Read the model definition and answer for the solid it produces. Units are mm, in the model's axes. Coordinates: 2 decimals unless noted, no trailing zeros. Write each loop counter-clockwise with the first axis right and the second up, starting at its lowest first coordinate (ties: lowest second). Pieces come first, ordered by that corner, then holes.
(1) The part is cut by section B-B, the plane y = 46. Determine the outline of the cut face in (x, z) (3 decimals).
(2) Straight lines are drawn through the part: line 1 along Z through (x, y) = (0.55, 61) (3 decimals); line 2 along Z through (x, y) = (1.45, 25.5); line 3 along Y through (x, z) = (2.9, 21). For each, find the intervals that lie inside material, in ascending order.
(3) The part is cut by section A-A, the plane y = 35. Determine the outline of the cut face in (x, z), and give its area (3 significant figures).
(4) Given pin 1 (1.5 mm diameter, centred on x = 2, z = 8.5, fed in from +Y); pin 2 (1 mm diameter, centred on x = 2.5, z = 187, fed in from -Y) (3 decimals); pin 3 (1.5 mm diameter, centred on x = 2, z = 198, fed in from -Y), each flat-ended and moving along its own axis, determine where each tip first touches the part or whether it passes through.
(5) The part is cut by section C-C, the plane x = 2.25. Determine the outline of the cut face in (y, z) (3 decimals).
(6) The part is cut by section D-D, the plane z = 59.5. Determine the outline of the cut face in (x, y).
Autodesk Inventor part; units mm, degrees
ref_plane "YZ Plane" through (0, 0, 0) normal (1, 0, 0) x (0, 1, 0)
ref_plane "XZ Plane" through (0, 0, 0) normal (0, 1, 0) x (-1, 0, 0)
ref_plane "XY Plane" through (0, 0, 0) normal (0, 0, 1) x (1, 0, 0)
sketch "Sketch1" plane through (0, 0, 0) normal (0, 0, 1) x (1, 0, 0)
  line L0 (25.4, 0) -> (146.304, 0)
  line L1 (171.704, 25.4) -> (171.704, 63.5)
  line L2 (171.704, 63.5) -> (0, 63.5)
  line L3 (0, 63.5) -> (0, 25.4)
  arc A0 (0, 25.4) -> (25.4, 0) centre (25.4, 25.4) ccw
  arc A1 (146.304, 0) -> (171.704, 25.4) centre (146.304, 25.4) ccw
  point P0 (0, 0)
  dimension "d0" = 171.704
  dimension "d2" = 50.8
  dimension "d3" = 50.8
  dimension "d4" = 63.5
  dimension "d5" = 63.5
  dimension "d6" = 0
extrude "Extrusion1" add sketch "Sketch1" along normal blind 304.8
sketch "Sketch2" plane through (0, 0, 304.8) normal (0, 0, 1) x (1, 0, 0)
  line L0 (25.4, 0) -> (146.304, 0)
  line L1 (3.048, 63.5) -> (206.248, 63.5)
  line L2 (206.248, 63.5) -> (206.248, 0)
  line L3 (206.248, 0) -> (3.048, 0)
  line L4 (3.048, 0) -> (3.048, 63.5)
  line L5 (171.704, 63.5) -> (0, 63.5)
  line L6 (0, 63.5) -> (0, 25.4)
  point P0 (0, 0)
  dimension "d9" = 0
  dimension "d10" = 203.2
  dimension "d11" = 3.048
extrude "Extrusion2" cut sketch "Sketch2" against normal through all
sketch "Sketch5" plane through (0, 25.4, 0) normal (-1, 0, 0) x (0, 0, 1)
  line L0 (6.985, 38.1) -> (10.033, 38.1)
  line L1 (10.033, 38.1) -> (10.033, 12.7)
  line L2 (10.033, 12.7) -> (6.985, 12.7)
  line L3 (6.985, 12.7) -> (6.985, 38.1)
  line L4 (0, 38.1) -> (304.8, 38.1)
  line L5 (0, 38.1) -> (0, 0)
  line L6 (152.4, 38.1) -> (152.4, 0)
  line L7 (0, 0) -> (304.8, 0)
  line L8 (297.815, 38.1) -> (294.767, 38.1)
  line L9 (294.767, 38.1) -> (294.767, 12.7)
  line L10 (294.767, 12.7) -> (297.815, 12.7)
  line L11 (297.815, 12.7) -> (297.815, 38.1)
  line L12 (304.8, 38.1) -> (0, 38.1)
  line L13 (304.8, 38.1) -> (304.8, 0)
  point P0 (0, -25.4)
  point P1 (297.815, 38.1)
  point P2 (294.767, 38.1)
  dimension "d22" = 3.048
  dimension "d23" = 25.4
  dimension "d24" = 0
  dimension "d25" = 6.985
extrude "Extrusion5" cut sketch "Sketch5" against normal through all contours L0 L1 L2 L3 | L4 L11 L10 L9
sketch "Sketch6" plane through (0, 25.4, 0) normal (-1, 0, 0) x (0, 0, 1)
  line L0 (10.033, 38.1) -> (294.767, 38.1)
  line L1 (0, 0) -> (304.8, 0)
  line L2 (35.433, 38.1) -> (269.367, 38.1)
  line L3 (269.367, 38.1) -> (269.367, 0)
  line L4 (269.367, 0) -> (35.433, 0)
  line L5 (35.433, 0) -> (35.433, 38.1)
  line L6 (10.033, 38.1) -> (10.033, 12.7)
  line L7 (294.767, 12.7) -> (294.767, 38.1)
  point P0 (0, -25.4)
  point P1 (35.433, 0)
  dimension "d28" = 25.4
  dimension "d29" = 25.4
extrude "Extrusion6" cut sketch "Sketch6" against normal through all
properties part number "Battery_container_side"
Computed:
1. outline: (0, 0) - (3.048, 0) - (3.048, 6.985) - (0, 6.985) - close; (0, 10.033) - (3.048, 10.033) - (3.048, 35.433) - (0, 35.433) - close; (0, 269.367) - (3.048, 269.367) - (3.048, 294.767) - (0, 294.767) - close; (0, 297.815) - (3.048, 297.815) - (3.048, 304.8) - (0, 304.8) - close
2. line 1: z = 0 to 6.985, 10.033 to 35.433, 269.367 to 294.767, 297.815 to 304.8
2. line 2: z = 0 to 35.43, 269.37 to 304.8
2. line 3: y = 13.61 to 63.5
3. outline: (0, 0) - (3.05, 0) - (3.05, 35.43) - (0, 35.43) - close; (0, 269.37) - (3.05, 269.37) - (3.05, 304.8) - (0, 304.8) - close
3. area: 216 mm2
4. pin 1: stops at y = 38.1
4. pin 2: stops at y = 13.425
4. pin 3: stops at y = 13.9
5. outline: (14.948, 0) - (63.5, 0) - (63.5, 6.985) - (38.1, 6.985) - (38.1, 10.033) - (63.5, 10.033) - (63.5, 35.433) - (25.4, 35.433) - (25.4, 269.367) - (63.5, 269.367) - (63.5, 294.767) - (38.1, 294.767) - (38.1, 297.815) - (63.5, 297.815) - (63.5, 304.8) - (14.948, 304.8) - close
6. outline: (0, 25.4) arc R25.4 ccw to (3.05, 13.34) - (3.05, 25.4) - close
